Source: CAD feature listing. Evaluate the final solid. Frame: model axes, mm. A direction names the side the tool comes from. Round coordinates to 2 decimals unless told otherwise and drop trailing zeros. Write each loop counter-clockwise with the first axis right and the second up, starting at its lowest first coordinate (ties: lowest second). Pieces come first, ordered by that corner, then holes.
from build123d import *

# Parameters (mm, degrees)
F0_W     = 38.1
F0_H     = 38.1
F6_DEPTH = 6.35
F1_R     = 3.175
F7_DEPTH = 6.35
F2_W     = 6.35
F2_H     = 3.175
F3_W     = 6.35
F3_H     = 3.175
F8_DEPTH = 6.35
F4_R     = 1.5875
F5_R     = 1.5875
F9_DEPTH = 19.05


with BuildPart() as f6:
    # F0 (on Front) → F6 (new body, symmetric)
    with BuildSketch(Plane.XZ):
        Rectangle(F0_W, F0_H)
    extrude(amount=F6_DEPTH, both=True)

    # F1 (on Front) → F7 (cut, symmetric)
    with BuildSketch(Plane.XZ):
        Circle(F1_R)
    extrude(amount=F7_DEPTH, both=True, mode=Mode.SUBTRACT)

    # F2 (on Front) + F3 (on Front) → F8 (cut, symmetric)
    with BuildSketch(Plane.XZ):
        with Locations((-15.875, -1.5875)):
            Rectangle(F2_W, F2_H)
    with BuildSketch(Plane.XZ):
        with Locations((15.875, -1.5875)):
            Rectangle(F3_W, F3_H)
    extrude(amount=F8_DEPTH, both=True, mode=Mode.SUBTRACT)

    # F4 (on Right) + F5 (on Right) → F9 (cut, symmetric)
    with BuildSketch(Plane.YZ):
        with Locations((0, 12.7)):
            Circle(F4_R)
    with BuildSketch(Plane.YZ):
        with Locations((0, -12.7)):
            Circle(F5_R)
    extrude(amount=F9_DEPTH, both=True, mode=Mode.SUBTRACT)


solid = f6.part
1) Section query A-A on x = -17. State how many separate pieces and enclosed holes the cut face has, then the cut area to 3 significant figures.
Taken from the geometry:
separate pieces: 2
enclosed holes: 2
area: 428 mm2
2) Material intervals for line 1 (Z direction, x = 7.75, y = 0); line 2 (Z direction, x = 0, y = -3) (3 decimals); line 3 (Z direction, x = -7, y = -0.5), sorted ascending.
Taken from the geometry:
line 1: z = -19.05 to -14.29, -11.11 to 11.11, 14.29 to 19.05
line 2: z = -19.05 to -3.175, 3.175 to 19.05
line 3: z = -19.05 to -14.21, -11.19 to 11.19, 14.21 to 19.05
3) Contact query for flat-ended pins moving along their axis: P1, Ø3.5, axis at y = -1.5, z = -1.5, coming from the +X side; P2, Ø2.5, axis at y = 2.5, z = -1.5, coming from the -X side. Output: stop coordinate, or through.
Taken from the geometry:
P1: stops at x = 19.05
P2: stops at x = -12.7
4) Section query D-D on y = 1. Return the cut outline in (x, z) (3 decimals).
Taken from the geometry:
outline: (-19.05, -19.05) - (19.05, -19.05) - (19.05, -13.933) - (-19.05, -13.933) - close; (-19.05, -11.467) - (19.05, -11.467) - (19.05, -3.175) - (12.7, -3.175) - (12.7, 0) - (19.05, 0) - (19.05, 11.467) - (-19.05, 11.467) - (-19.05, 0) - (-12.7, 0) - (-12.7, -3.175) - (-19.05, -3.175) - close; (-19.05, 13.933) - (19.05, 13.933) - (19.05, 19.05) - (-19.05, 19.05) - close; hole circle Ø6.35 at (0, 0)
5) Section query B-B on z = -12.7. Return the cut outline in (x, y), then the cut area to 3 significant figures.
Taken from the geometry:
outline: (-19.05, -6.35) - (19.05, -6.35) - (19.05, -1.59) - (-19.05, -1.59) - close; (-19.05, 1.59) - (19.05, 1.59) - (19.05, 6.35) - (-19.05, 6.35) - close
area: 363 mm2
6) Section query C-C on y = 3.5. Return the cut outline in (x, z) (3 decimals), then the cut area to 3 significant figures.
Taken from the geometry:
outline: (-19.05, -19.05) - (19.05, -19.05) - (19.05, -3.175) - (12.7, -3.175) - (12.7, 0) - (19.05, 0) - (19.05, 19.05) - (-19.05, 19.05) - (-19.05, 0) - (-12.7, 0) - (-12.7, -3.175) - (-19.05, -3.175) - close; hole circle Ø6.35 at (0, 0)
area: 1,380 mm2
7) Reachability of faces 1 (the face through (16, 0, -3.175)), 2 (the face through (4, -6.35, 0)), 3 (the face through (-12.7, 0, -2)) from +Z, -Z, +X, -X, +Y, -Y: full face, straight path, thin tool, end or side. Return the list, or none.
Taken from the geometry:
face 1: +X, +Y, -Y
face 2: +Z, -Z, +X, -X, -Y
face 3: -X, +Y, -Y
8) Pull-direction query (Z, two-part tool) for faces 4 (the face through (-19.05, 0, 9)), 5 (the face through (16, 0, 0)), 6 (the face through (0, 0, -19.05)); classes: released by +Z, released by -Z, zero draft, split by the parting line, or undercut.
Taken from the geometry:
face 4: zero draft
face 5: undercut
face 6: released by -Z
